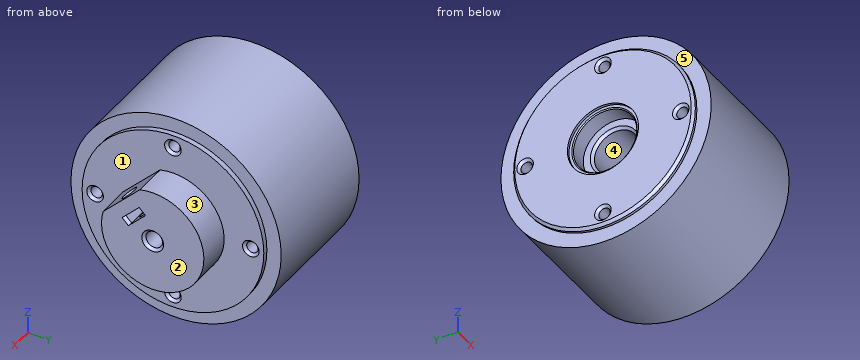
```python
from build123d import *

# Parameters (mm, degrees)
SKETCH012_R     = 40.5
PAD008_DEPTH    = 25
SKETCH015_R     = 35
PAD011_DEPTH    = 2
SKETCH016_R     = 2.2
POCKET003_DEPTH = 54.001
PAD013_DEPTH    = 13
SKETCH020_R     = 3.2
POCKET004_DEPTH = 67.001
SKETCH019_R     = 2.1
POCKET005_DEPTH = 17
POCKET006_DEPTH = 9
CHAMFER025_SIZE = 1
CHAMFER026_SIZE = 0.4
CHAMFER034_SIZE = 1
CHAMFER035_SIZE = 1


with BuildPart() as part:
    # Sketch012 → Pad008 (new body, symmetric)
    with BuildSketch(Plane.YZ):
        Circle(SKETCH012_R)
    extrude(amount=PAD008_DEPTH, both=True)

    # Sketch015 (on Face3 of Pad008) → Pad011 (join)
    with BuildSketch(Plane.YZ.offset(25)):
        Circle(SKETCH015_R)
    pad011 = extrude(amount=PAD011_DEPTH)

    # Mirrored001: Pad011 across YZ
    add(pad011.mirror(Plane.YZ))

    # Sketch016 (on Face7 of Mirrored001) → Pocket003 (cut, through all)
    with BuildSketch(Plane.YZ.offset(27)):
        with Locations((0, 30)):
            Circle(SKETCH016_R)
        with Locations((-30, 0)):
            Circle(SKETCH016_R)
        with Locations((0, -30)):
            Circle(SKETCH016_R)
        with Locations((30, 0)):
            Circle(SKETCH016_R)
    extrude(amount=-POCKET003_DEPTH, mode=Mode.SUBTRACT)

    # Sketch018 (on Face7 of Pocket003) → Pad013 (join)
    with BuildSketch(Plane.YZ.offset(27)):
        with BuildLine():
            ThreePointArc((-19.091883, 4.949747), (13.946326, -13.946326), (-4.949747, 19.091883))
            Line((-19.091883, 4.949747), (-4.949747, 19.091883))
        make_face()
    extrude(amount=PAD013_DEPTH)

    # Sketch020 (on Face14 of Pad013) → Pocket004 (cut, through all)
    with BuildSketch(Plane.YZ.offset(40)):
        Circle(SKETCH020_R)
    extrude(amount=-POCKET004_DEPTH, mode=Mode.SUBTRACT)

    # Sketch019 (on Face13 of Pad013) → Pocket005 (cut)
    with BuildSketch(Plane(origin=(0, -12.020815, 12.020815), x_dir=(1, 0, 0), z_dir=(0, -0.707107, 0.707107))):
        with Locations((35, 0)):
            Circle(SKETCH019_R)
    extrude(amount=-POCKET005_DEPTH, mode=Mode.SUBTRACT)

    # Sketch021 (on Face15 of Pocket005) → Pocket006 (cut)
    with BuildSketch(Plane.YZ.offset(40)):
        Polygon((-11.066221, 5.904342), (-8.662058, 3.500179), (-3.500179, 8.662058), (-5.904342, 11.066221), align=None)
    extrude(amount=-POCKET006_DEPTH, mode=Mode.SUBTRACT)

    # Sketch067 → Groove (revolve, cut)
    with BuildSketch(Plane.XZ):
        Polygon((-27.5, 0), (-27.5, 13.7), (-26, 13.7), (-26, 12.2), (-19.3, 12.2), (-19.3, 8.5), (0, 8.5), (0, 0), align=None)
    revolve(axis=Axis((0, 0, 0), (1, 0, 0)), mode=Mode.SUBTRACT)

    # Chamfer025
    chamfer025_edges = [part.edges().sort_by_distance(p)[0] for p in [
        (-19.3, 0, -8.5),
    ]]
    chamfer(chamfer025_edges, length=CHAMFER025_SIZE)

    # Chamfer026
    chamfer026_edges = [part.edges().sort_by_distance(p)[0] for p in [
        (-26, 0, -12.2),
    ]]
    chamfer(chamfer026_edges, length=CHAMFER026_SIZE)

    # Chamfer034
    chamfer034_edges = [part.edges().sort_by_distance(p)[0] for p in [
        (-27, 27.8, 0),
        (-27, -2.2, 30),
        (-27, -32.2, 0),
        (-27, -2.2, -30),
        (27, -32.2, 0),
        (27, -2.2, -30),
        (27, 27.8, 0),
        (27, -2.2, 30),
        (-27, -35, 0),
    ]]
    chamfer(chamfer034_edges, length=CHAMFER034_SIZE)

    # Chamfer035
    chamfer035_edges = [part.edges().sort_by_distance(p)[0] for p in [
        (40, -3.2, 0),
        (32.9, -12.020815, 12.020815),
        (40, -9.86414, 4.70226),
        (40, -4.70226, 9.86414),
    ]]
    chamfer(chamfer035_edges, length=CHAMFER035_SIZE)


solid = part.part
```
Input: part model. Units: mm. Frame: model coordinates. Face numbers are marked on the shaded views. A direction names the side the tool comes from. Give positions to 0.01 mm unless a question says otherwise; leave off trailing zeros. Order: outer loops, then holes, each group sorted by start corner. A loop starts at its lowest first (then second) coordinate and runs counter-clockwise, first axis right, second up. Notation, with made-up numbers: M -30,-1.5 L -18,-1.5 A24 cw -18,30.5 Z; hole C 58.25,38 d4. An arc over 180 degrees is marked long. One line per question, with ' | ' between items. Start each with the question number.
1. Pull-direction query (Y, two-part tool) for the marked faces 3, 4 and 5; classes: released by +Y, released by -Y, zero draft, split by the parting line, or undercut.
2. Material intervals for probe 1 along Z at (x, y) = (-6, 0); probe 2 along Z at (x, y) = (23.5, -0.5); probe 3 along X at (y, z) = (21, -14.5), sorted ascending. Write a range as [from, to].
3. Section query A-A (x = -11). Return the cut outline in (y, z), and give its area (3 significant figures).
4. Section query B-B (x = 15). Return the cut outline in (y, z).
5. First-contact query: pin 1 Ø12 at (x, z) = (-18, 23.5) entering from +Y; pin 2 Ø5 at (y, z) = (3, 28.5) entering from +X; pin 3 Ø4 at (x, z) = (5, -13.5) entering from +Y; pin 4 Ø8.5 at (y, z) = (-5.5, 7.5) entering from +X. Flat tips, straight axial feed; report the tip coordinate or a pass-through.
6. Access query for the marked faces 1 and 2. Directions: +Z, -Z, +X, -X, +Y, -Y. A direction counts if a zero-diameter tool reaches every point of the face in a straight line with its end or side. Return the directions, or none.
Here are the results:
1) face 3: split by the parting line | face 4: undercut | face 5: zero draft
2) probe 1: [-40.5, -32.2], [-27.8, -8.5], [8.5, 27.8], [32.2, 40.5] | probe 2: [-40.5, -32.14], [-27.86, -3.16], [3.16, 27.86], [32.14, 40.5] | probe 3: [-27, 27]
3) outline: C 0,0 d81; hole C -30,0 d4.4; hole C 0,0 d17; hole C 0,-30 d4.4; hole C 0,30 d4.4; hole C 30,0 d4.4 | area: 4,870 mm²
4) outline: C 0,0 d81; hole C -30,0 d4.4; hole C 0,0 d6.4; hole C 0,-30 d4.4; hole C 0,30 d4.4; hole C 30,0 d4.4
5) pin 1: y = 36.52 | pin 2: x = 27 | pin 3: y = 38.83 | pin 4: x = 40
6) face 1: +X | face 2: +Z, -Z, +X, +Y, -Y
